from build123d import *

# Parameters (mm, degrees)
F1_DEPTH = 25.4


with BuildPart() as f1:
    # F0 (on Top) → F1 (new body)
    with BuildSketch(Plane.XY):
        with BuildLine():
            ThreePointArc((29.598609, 7.333415), (27.189668, 12.904555), (23.743974, 17.901333))
            ThreePointArc((23.743974, 17.901333), (18.4404, 22.863979), (12.12993, 26.460327))
            ThreePointArc((12.12993, 26.460327), (-0.552402, 28.919903), (-13.139316, 26.011181))
            ThreePointArc((-13.139316, 26.011181), (-23.690129, 17.964895), (-29.92398, 6.251592))
            ThreePointArc((-29.92398, 6.251592), (-31.002085, 0.087719), (-30.823785, -6.167186))
            ThreePointArc((-30.823785, -6.167186), (-28.826395, -13.786695), (-24.977811, -20.659459))
            ThreePointArc((-24.977811, -20.659459), (-20.502768, -25.521151), (-15.101192, -29.327071))
            ThreePointArc((-15.101192, -29.327071), (-7.516447, -32.319411), (0.585505, -33.236383))
            ThreePointArc((0.585505, -33.236383), (7.228176, -32.389792), (13.535374, -30.140119))
            ThreePointArc((13.535374, -30.140119), (20.27418, -25.719795), (25.650061, -19.715574))
            ThreePointArc((25.650061, -19.715574), (28.724195, -14.036908), (30.55867, -7.845603))
            ThreePointArc((30.55867, -7.845603), (30.951906, -5.014149), (31.083355, -2.158543))
            ThreePointArc((31.083355, -2.158543), (30.709925, 2.645147), (29.598609, 7.333415))
        make_face()
        with BuildLine():
            ThreePointArc((12.12993, 26.460327), (18.4404, 22.863979), (23.743974, 17.901333))
            Line((23.743974, 17.901333), (43.890379, 33.241566))
            Line((43.890379, 33.241566), (23.743974, 51.085521))
            Line((23.743974, 51.085521), (12.12993, 26.460327))
        make_face()
        with BuildLine():
            Line((54.744394, 13.287515), (29.598609, 7.333415))
            ThreePointArc((29.598609, 7.333415), (30.709925, 2.645147), (31.083355, -2.158543))
            ThreePointArc((31.083355, -2.158543), (30.951906, -5.014149), (30.55867, -7.845603))
            Line((30.55867, -7.845603), (53.354507, -13.589103))
            Line((53.354507, -13.589103), (54.744394, 13.287515))
        make_face()
        with BuildLine():
            ThreePointArc((-24.977811, -20.659459), (-28.826395, -13.786695), (-30.823785, -6.167186))
            Line((-30.823785, -6.167186), (-53.96684, -10.906294))
            Line((-53.96684, -10.906294), (-43.557758, -35.724339))
            Line((-43.557758, -35.724339), (-24.977811, -20.659459))
        make_face()
        with BuildLine():
            Line((44.521169, -34.516261), (25.650061, -19.715574))
            ThreePointArc((25.650061, -19.715574), (20.27418, -25.719795), (13.535374, -30.140119))
            Line((13.535374, -30.140119), (22.641603, -50.1869))
            Line((22.641603, -50.1869), (44.521169, -34.516261))
        make_face()
        with BuildLine():
            ThreePointArc((0.585505, -33.236383), (-7.516447, -32.319411), (-15.101192, -29.327071))
            Line((-15.101192, -29.327071), (-25.12089, -48.992938))
            Line((-25.12089, -48.992938), (0.772595, -56.328588))
            Line((0.772595, -56.328588), (0.585505, -33.236383))
        make_face()
    extrude(amount=F1_DEPTH)


solid = f1.part
Design review of the part built by this model. Coordinates are the model's own, in mm. A direction names the side the tool comes from. Coordinates: 2 decimals unless noted, no trailing zeros. Loops run counter-clockwise (first coordinate to the right, second up) from the corner with the lowest first, then second, coordinate; pieces in that order, holes last.
Item 1: Add section A-A (z = 23.75). Write out the cut boundary in (x, y), and give its area (3 significant figures).
Completed:
outline: (-53.97, -10.91) - (-43.56, -35.72) - (-24.98, -20.66) arc R31.08 ccw to (-15.1, -29.33) - (-25.12, -48.99) - (0.77, -56.33) - (0.59, -33.24) arc R31.08 ccw to (13.54, -30.14) - (22.64, -50.19) - (44.52, -34.52) - (25.65, -19.72) arc R31.08 ccw to (30.56, -7.85) - (53.35, -13.59) - (54.74, 13.29) - (29.6, 7.33) arc R31.08 ccw to (23.74, 17.9) - (43.89, 33.24) - (23.74, 51.09) - (12.13, 26.46) arc R31.08 ccw to (-29.92, 6.25) arc R31.08 ccw to (-30.82, -6.17) - close
area: 5,460 mm2
Item 2: Add section B-B (x = 28). Write out the cut boundary in (y, z), and give its area (3 significant figures).
Completed:
outline: (-46.35, 0) - (-21.56, 0) - (-21.56, 25.4) - (-46.35, 25.4) - close; (-15.66, 0) - (11.34, 0) - (11.34, 25.4) - (-15.66, 25.4) - close; (21.14, 0) - (47.32, 0) - (47.32, 25.4) - (21.14, 25.4) - close
area: 1,980 mm2
Item 3: Clearance check with flat-ended pins moving along their axes: pin 1 (3 mm diameter, centred on y = -10.5, z = 20, fed in from +X); pin 2 (3 mm diameter, centred on y = -9, z = 9, fed in from +X); pin 3 (4 mm diameter, centred on y = 38.5, z = 19.5, fed in from +X). State where each tip first meets the part, or that it passes through.
Completed:
pin 1: stops at x = 53.59
pin 2: stops at x = 53.67
pin 3: stops at x = 40.21
Item 4: Add section D-D (x = -18). Write out the cut boundary in (y, z), and give its area (3 significant figures).
Completed:
outline: (-51.01, 0) - (-35.02, 0) - (-35.02, 25.4) - (-51.01, 25.4) - close; (-27.5, 0) - (23.18, 0) - (23.18, 25.4) - (-27.5, 25.4) - close
area: 1,690 mm2
Item 5: For faces 4 (the flat face through (35.22, -27.22, 12.52)), 5 (the flat face through (-48.835, -23.142, 12.522)), 6 (the flat face through (41.797, -10.677, 12.522)), 7 (the flat face through (33.43, -42.46, 12.52)), 8 (the flat face through (18.025, -40.023, 12.522)), list the 3-axis set-ups (+Z, -Z, +X, -X, +Y, -Y) from which the entire face can be reached by the end or side of a thin tool; tool diameter is ignored.
Completed:
face 4: +Z, -Z, +X
face 5: +Z, -Z, -X, -Y
face 6: +Z, -Z
face 7: +Z, -Z, +X, -Y
face 8: +Z, -Z, -Y
Item 6: Add section C-C (y = -46.5). Write out the cut boundary in (x, z).
Completed:
outline: (-23.85, 0) - (0.69, 0) - (0.69, 25.4) - (-23.85, 25.4) - close; (20.97, 0) - (27.79, 0) - (27.79, 25.4) - (20.97, 25.4) - close
Item 7: Wall thickness on L1, parallel to Y at x = 34, z = 8.75; L2, parallel to X at y = -39, z = 23.5; L3, parallel to Y at x = -41, z = 6: over which ranges is each line inside the solid? List them lowest first.
Completed:
L1: y = -42.05 to -26.26, -8.71 to 8.38, 25.71 to 42
L2: x = -20.03 to 0.63, 17.56 to 38.26
L3: y = -33.65 to -8.25
Item 8: Draft analysis for pull direction X (two halves, no side actions). For faces 1 (the cylindrical face through (-30.996, 0.175, 12.522)), 2 (the cylindrical face through (27.23, 12.83, 12.52)), 3 (the flat face through (54.04, -0.34, 12.52)), state which applies: pulls with the +X half, pulls with the -X half, needs draft (parallel to the pull), parting line crosses it, or undercut.
Completed:
face 1: pulls with the -X half
face 2: undercut
face 3: pulls with the +X half
